Source: CAD feature listing. Evaluate the final solid. Frame: model axes, mm. Face numbers are marked on the shaded views. A direction names the side the tool comes from. Round coordinates to 2 decimals unless told otherwise and drop trailing zeros. Loops run counter-clockwise (first coordinate to the right, second up) from the corner with the lowest first, then second, coordinate; pieces in that order, holes last. Notation, with made-up numbers: (42.5, -28.5) -> (95.5, -28.5) arc R28 ccw to (95.5, -6.5) -> close; hole circle Ø11 at (60.5, -18.75). An arc over 180 degrees is marked (long way). Put each result on its own line as item: value. Start each with the question number.
1. Contact query for a flat-ended pin moving along its axis: pin 1 (1.5 mm diameter, centred on y = 3, z = -18, fed in from +X). Output: stop coordinate, or through.
2. Material intervals for L1, parallel to X at y = 4.35, z = 0; L2, parallel to Z at x = -22.25, y = 4; L3, parallel to Z at x = -6, y = 1.25, sorted ascending.
3. Draft query along Z for the marked faces 1, 2, 3 and 4. Return one class per face: pulls with the +Z half, pulls with the -Z half, needs draft (parallel to the pull), parting line crosses it, or undercut.
4. Cut plane A-A (x = 22.25). Return the cut outline in (y, z), then the cut area to 3 significant figures.
5. Cut plane B-B (z = 0). Return the cut outline in (x, y), then the cut area to 3 significant figures.
6. Cut plane C-C (y = 1.25). Return the cut outline in (x, z).
7. Cut plane D-D (x = -11.5). Return the cut outline in (y, z).
8. Set-up query: the marked faces 5 and 6. Return all of +Z, -Z, +X, -X, +Y, -Y with unobstructed straight access to the full face (end or side cutting, diameter ignored); none if empty.
```python
from build123d import *

# Parameters (mm, degrees)
SKETCH1_W            = 33.75
SKETCH1_H            = 50.4
SKETCH1_R            = 1.5
SKETCH1_W_2          = 20
SKETCH1_H_2          = 6.4
BOSS_EXTRUDE1_DEPTH  = 6
FILLET1_R            = 10
FILLET1_OF_MIRROR1_R = 10


with BuildPart() as part:
    # Sketch1 → Boss-Extrude1 (new body)
    with BuildSketch(Plane(origin=(0, 0, 0), x_dir=(1, 0, 0), z_dir=(0, 1, 0))):
        with Locations((-16.875, 0)):
            Rectangle(SKETCH1_W, SKETCH1_H)
        with Locations(Location((-22.25, 0, 0), (0, 0, 90))):
            Circle(SKETCH1_R, mode=Mode.SUBTRACT)
        with Locations((-13.75, 12)):
            Rectangle(SKETCH1_W_2, SKETCH1_H_2, mode=Mode.SUBTRACT)
        with Locations((-13.75, -12)):
            Rectangle(SKETCH1_W_2, SKETCH1_H_2, mode=Mode.SUBTRACT)
    boss_extrude1 = extrude(amount=BOSS_EXTRUDE1_DEPTH)

    # Fillet1
    fillet1_edges = [part.edges().sort_by_distance(p)[0] for p in [
        (-33.75, 3, -25.2),
        (-33.75, 3, 25.2),
    ]]
    fillet(fillet1_edges, radius=FILLET1_R)

    # Mirror1: Boss-Extrude1 across plane
    add(boss_extrude1.mirror(Plane(origin=(0, 6, -25.2), x_dir=(0, 0, 1), z_dir=(-1, 0, 0))))

    # Fillet1 of Mirror1
    fillet1_of_mirror1_edges = [part.edges().sort_by_distance(p)[0] for p in [
        (33.75, 3, -25.2),
        (33.75, 3, 25.2),
    ]]
    fillet(fillet1_of_mirror1_edges, radius=FILLET1_OF_MIRROR1_R)


solid = part.part
```
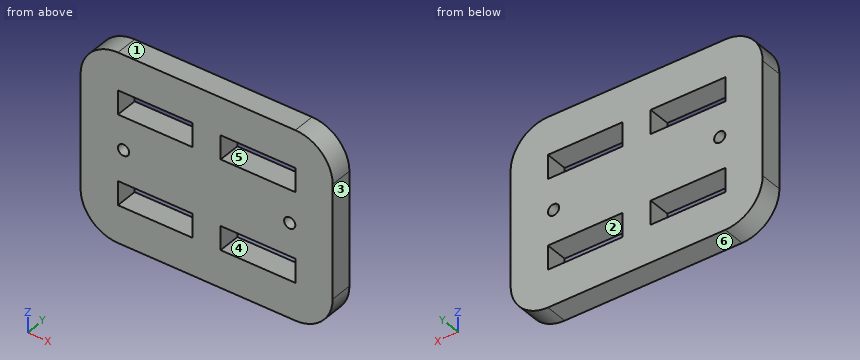
Solution:
1. pin 1: stops at x = 33.54
2. L1: x = -33.75 to -23.75, -20.75 to 20.75, 23.75 to 33.75
2. L2: z = -25.2 to -15.2, -8.8 to -1.5, 1.5 to 8.8, 15.2 to 25.2
2. L3: z = -25.2 to -15.2, -8.8 to 8.8, 15.2 to 25.2
3. face 1: pulls with the +Z half
3. face 2: undercut
3. face 3: needs draft
3. face 4: undercut
4. outline: (0, -25.2) -> (6, -25.2) -> (6, -15.2) -> (0, -15.2) -> close; (0, -8.8) -> (6, -8.8) -> (6, -1.5) -> (0, -1.5) -> close; (0, 1.5) -> (6, 1.5) -> (6, 8.8) -> (0, 8.8) -> close; (0, 15.2) -> (6, 15.2) -> (6, 25.2) -> (0, 25.2) -> close
4. area: 208 mm^2
5. outline: (-33.75, 0) -> (-23.75, 0) -> (-23.75, 6) -> (-33.75, 6) -> close; (-20.75, 0) -> (20.75, 0) -> (20.75, 6) -> (-20.75, 6) -> close; (23.75, 0) -> (33.75, 0) -> (33.75, 6) -> (23.75, 6) -> close
5. area: 369 mm^2
6. outline: (-33.75, -15.2) arc R10 ccw to (-23.75, -25.2) -> (23.75, -25.2) arc R10 ccw to (33.75, -15.2) -> (33.75, 15.2) arc R10 ccw to (23.75, 25.2) -> (-23.75, 25.2) arc R10 ccw to (-33.75, 15.2) -> close; hole (-23.75, -15.2) -> (-3.75, -15.2) -> (-3.75, -8.8) -> (-23.75, -8.8) -> close; hole circle Ø3 at (-22.25, 0); hole (-23.75, 8.8) -> (-3.75, 8.8) -> (-3.75, 15.2) -> (-23.75, 15.2) -> close; hole (3.75, -15.2) -> (23.75, -15.2) -> (23.75, -8.8) -> (3.75, -8.8) -> close; hole (3.75, 8.8) -> (23.75, 8.8) -> (23.75, 15.2) -> (3.75, 15.2) -> close; hole circle Ø3 at (22.25, 0)
7. outline: (0, -25.2) -> (6, -25.2) -> (6, -15.2) -> (0, -15.2) -> close; (0, -8.8) -> (6, -8.8) -> (6, 8.8) -> (0, 8.8) -> close; (0, 15.2) -> (6, 15.2) -> (6, 25.2) -> (0, 25.2) -> close
8. face 5: +Y, -Y
8. face 6: -Z, +X, -X, +Y, -Y
